The listing builds one solid part. Answer for the finished solid, in the listing's coordinates (mm). A direction names the side the tool comes from. Give positions to 0.01 mm unless a question says otherwise; leave off trailing zeros. Write each loop counter-clockwise with the first axis right and the second up, starting at its lowest first coordinate (ties: lowest second). Pieces come first, ordered by that corner, then holes. Notation, with made-up numbers: (-6.5, 7.25) -> (9.5, 7.25) arc R15 ccw to (9.5, 26.25) -> close; hole circle Ø9 at (-0.5, 88.5). An arc over 180 degrees is marked (long way). Put each result on its own line as item: value. Start each with the question number.
1) A flat-ended cylindrical pin translates along its axis: pin 1 Ø0.6 at (y, z) = (-0.5, -2) entering from +X. Find the tip coordinate at first contact, or state that the pin passes through.
2) A cutting plane is placed at A-A (y = 1.75). Give the number of separate pieces and of enclosed holes in the cut face, then the cut area to 3 significant figures.
3) For faces 1 (the flat face through (2, 2, -1.78)), 2 (the flat face through (2.4, 4.6, -0.9)), 3 (the flat face through (2, 0, -1)), determine the directions among +Z, -Z, +X, -X, +Y, -Y from which every point of the face is accessible in a straight line to the end or side of a thin tool.
4) A cutting plane is placed at B-B (x = 3.07). Write down the section's boundary in (y, z), then the cut area to 3 significant figures.
5) Find the intervals of material crossed by line 1 along Z through (x, y) = (0.8, 2); line 2 along Z through (x, y) = (3.8, 1.25); line 3 along Y through (x, z) = (4.2, -0.3), in increasing order. Write a range as from..to.
from build123d import *

# Parameters (mm, degrees)
SKETCH2_W           = 4.86
SKETCH2_H           = 1.78
BOSS_EXTRUDE1_DEPTH = 4.6
SKETCH3_R           = 0.22
CUT_EXTRUDE1_DEPTH  = 4.5
SKETCH4_W           = 0.2
SKETCH4_H           = 0.06
BOSS_EXTRUDE2_DEPTH = 1.96
SKETCH6_W           = 0.2
SKETCH6_H           = 0.06
BOSS_EXTRUDE3_DEPTH = 0.69
SKETCH7_W           = 0.2
SKETCH7_H           = 0.06
BOSS_EXTRUDE4_DEPTH = 2.4
SKETCH8_W           = 0.2
SKETCH8_H           = 0.06
BOSS_EXTRUDE5_DEPTH = 3.16


with BuildPart() as part:
    # Sketch2 → Boss-Extrude1 (new body)
    with BuildSketch(Plane(origin=(0, 0, 0), x_dir=(1, 0, 0), z_dir=(0, 1, 0))):
        with Locations((2.43, 0.89)):
            Rectangle(SKETCH2_W, SKETCH2_H)
    extrude(amount=BOSS_EXTRUDE1_DEPTH)

    # Sketch3 → Cut-Extrude1 (cut)
    with BuildSketch(Plane(origin=(0, 4.6, 0), x_dir=(1, 0, 0), z_dir=(0, 1, 0))):
        with Locations(Location((0.51, 1.27, 0), (0, 0, 270))):
            Circle(SKETCH3_R)
        with Locations(Location((1.15, 1.27, 0), (0, 0, 270))):
            Circle(SKETCH3_R)
        with Locations(Location((1.79, 1.27, 0), (0, 0, 270))):
            Circle(SKETCH3_R)
        with Locations(Location((2.43, 1.27, 0), (0, 0, 270))):
            Circle(SKETCH3_R)
        with Locations(Location((3.07, 1.27, 0), (0, 0, 270))):
            Circle(SKETCH3_R)
        with Locations(Location((3.71, 1.27, 0), (0, 0, 270))):
            Circle(SKETCH3_R)
        with Locations(Location((4.35, 1.27, 0), (0, 0, 270))):
            Circle(SKETCH3_R)
        with Locations(Location((1.15, 0.51, 0), (0, 0, 270))):
            Circle(SKETCH3_R)
        with Locations(Location((1.79, 0.51, 0), (0, 0, 270))):
            Circle(SKETCH3_R)
        with Locations(Location((2.43, 0.51, 0), (0, 0, 270))):
            Circle(SKETCH3_R)
        with Locations(Location((3.07, 0.51, 0), (0, 0, 270))):
            Circle(SKETCH3_R)
        with Locations(Location((3.71, 0.51, 0), (0, 0, 270))):
            Circle(SKETCH3_R)
        with Locations(Location((4.35, 0.51, 0), (0, 0, 270))):
            Circle(SKETCH3_R)
        with Locations(Location((0.51, 0.51, 0), (0, 0, 270))):
            Circle(SKETCH3_R)
    extrude(amount=-CUT_EXTRUDE1_DEPTH, mode=Mode.SUBTRACT)

    # Sketch4 → Boss-Extrude2 (add)
    with BuildSketch(Plane.XZ):
        with Locations((0.51, -0.51)):
            Rectangle(SKETCH4_W, SKETCH4_H)
        with Locations((1.15, -0.51)):
            Rectangle(SKETCH4_W, SKETCH4_H)
        with Locations((1.79, -0.51)):
            Rectangle(SKETCH4_W, SKETCH4_H)
        with Locations((2.43, -0.51)):
            Rectangle(SKETCH4_W, SKETCH4_H)
        with Locations((3.07, -0.51)):
            Rectangle(SKETCH4_W, SKETCH4_H)
        with Locations((3.71, -0.51)):
            Rectangle(SKETCH4_W, SKETCH4_H)
        with Locations((4.35, -0.51)):
            Rectangle(SKETCH4_W, SKETCH4_H)
    extrude(amount=BOSS_EXTRUDE2_DEPTH)

    # Sketch6 → Boss-Extrude3 (add)
    with BuildSketch(Plane.XZ):
        with Locations((0.51, -1.27)):
            Rectangle(SKETCH6_W, SKETCH6_H)
        with Locations((1.15, -1.27)):
            Rectangle(SKETCH6_W, SKETCH6_H)
        with Locations((1.79, -1.27)):
            Rectangle(SKETCH6_W, SKETCH6_H)
        with Locations((2.43, -1.27)):
            Rectangle(SKETCH6_W, SKETCH6_H)
        with Locations((3.07, -1.27)):
            Rectangle(SKETCH6_W, SKETCH6_H)
        with Locations((3.71, -1.27)):
            Rectangle(SKETCH6_W, SKETCH6_H)
        with Locations((4.35, -1.27)):
            Rectangle(SKETCH6_W, SKETCH6_H)
    extrude(amount=BOSS_EXTRUDE3_DEPTH)

    # Sketch7 → Boss-Extrude4 (add)
    with BuildSketch(Plane(origin=(0, 0, -1.3), x_dir=(-1, 0, 0), z_dir=(0, 0, -1))):
        with Locations((-4.35, -0.66)):
            Rectangle(SKETCH7_W, SKETCH7_H)
        with Locations((-3.71, -0.66)):
            Rectangle(SKETCH7_W, SKETCH7_H)
        with Locations((-3.07, -0.66)):
            Rectangle(SKETCH7_W, SKETCH7_H)
        with Locations((-2.43, -0.66)):
            Rectangle(SKETCH7_W, SKETCH7_H)
        with Locations((-1.79, -0.66)):
            Rectangle(SKETCH7_W, SKETCH7_H)
        with Locations((-1.15, -0.66)):
            Rectangle(SKETCH7_W, SKETCH7_H)
        with Locations((-0.51, -0.66)):
            Rectangle(SKETCH7_W, SKETCH7_H)
    extrude(amount=BOSS_EXTRUDE4_DEPTH)

    # Sketch8 → Boss-Extrude5 (add)
    with BuildSketch(Plane(origin=(0, 0, -0.54), x_dir=(-1, 0, 0), z_dir=(0, 0, -1))):
        with Locations((-4.35, -1.93)):
            Rectangle(SKETCH8_W, SKETCH8_H)
        with Locations((-3.71, -1.93)):
            Rectangle(SKETCH8_W, SKETCH8_H)
        with Locations((-3.07, -1.93)):
            Rectangle(SKETCH8_W, SKETCH8_H)
        with Locations((-2.43, -1.93)):
            Rectangle(SKETCH8_W, SKETCH8_H)
        with Locations((-1.79, -1.93)):
            Rectangle(SKETCH8_W, SKETCH8_H)
        with Locations((-1.15, -1.93)):
            Rectangle(SKETCH8_W, SKETCH8_H)
        with Locations((-0.51, -1.93)):
            Rectangle(SKETCH8_W, SKETCH8_H)
    extrude(amount=BOSS_EXTRUDE5_DEPTH)


solid = part.part
Reply:
1. pin 1: stops at x = 4.45
2. separate pieces: 1
2. enclosed holes: 14
2. area: 6.52 mm2
3. face 1: -Z, +X, -X, +Y
3. face 2: +Z, -Z, +X, -X, +Y
3. face 3: none
4. outline: (-1.96, -3.7) -> (-1.9, -3.7) -> (-1.9, -0.54) -> (0, -0.54) -> (0, -1.24) -> (-0.69, -1.24) -> (-0.69, -3.7) -> (-0.63, -3.7) -> (-0.63, -1.3) -> (0, -1.3) -> (0, -1.78) -> (4.6, -1.78) -> (4.6, -1.49) -> (0.1, -1.49) -> (0.1, -1.05) -> (4.6, -1.05) -> (4.6, -0.73) -> (0.1, -0.73) -> (0.1, -0.29) -> (4.6, -0.29) -> (4.6, 0) -> (0, 0) -> (0, -0.48) -> (-1.96, -0.48) -> close
4. area: 4.72 mm2
5. line 1: z = -1.78..0
5. line 2: z = -1.78..-1.47, -1.07..-0.71, -0.31..0
5. line 3: y = 0..4.6
